from build123d import *

# Parameters (mm, degrees)
F0_W     = 10
F0_H     = 31
F0_R     = 1.8
F1_DEPTH = 4
F0_H_2   = 3
F2_DEPTH = 19
F3_R     = 1.8
F4_DEPTH = 25
F5_R     = 2


with BuildPart() as f1:
    # F0 (on Front) → F1 (new body)
    with BuildSketch(Plane.XZ):
        with Locations((0.497756, 2.022149)):
            Rectangle(F0_W, F0_H)
        with Locations((0.497756, 13.522149)):
            Circle(F0_R, mode=Mode.SUBTRACT)
    extrude(amount=F1_DEPTH)

    # F0 (on Front) → F2 (join)
    with BuildSketch(Plane.XZ):
        with Locations((0.497756, -14.977851)):
            Rectangle(F0_W, F0_H_2)
    extrude(amount=F2_DEPTH)

    # F3 (on face) → F4 (cut)
    with BuildSketch(Plane.XY.offset(-13.477851)):
        with Locations((0.497756, -14)):
            Circle(F3_R)
    extrude(amount=-F4_DEPTH, mode=Mode.SUBTRACT)

    # F5
    f5_edges = [f1.edges().sort_by_distance(p)[0] for p in [
        (-4.502244, -2, 17.522149),
        (5.497756, -2, 17.522149),
        (5.497756, -19, -14.977851),
        (-4.502244, -19, -14.977851),
    ]]
    fillet(f5_edges, radius=F5_R)


solid = f1.part
Work out the finished part from the listing and answer in its coordinate system (mm). A direction names the side the tool comes from. Give positions to 0.01 mm unless a question says otherwise; leave off trailing zeros. Loops run counter-clockwise (first coordinate to the right, second up) from the corner with the lowest first, then second, coordinate; pieces in that order, holes last. Notation, with made-up numbers: M 52.5,48.25 L 80.5,48.25 A21 ccw 80.5,73.25 Z; hole C 54.25,76 d6. An arc over 180 degrees is marked long. Use CSV: the item, a comma, the result in double quotes.
1) Find section A-A on y = -14. Write down the section's boundary in (x, z), plus the area to 3 significant figures.
Answer:
outline,"M -4.5,-16.48 L -1.3,-16.48 L -1.3,-13.48 L -4.5,-13.48 Z; M 2.3,-16.48 L 5.5,-16.48 L 5.5,-13.48 L 2.3,-13.48 Z"
area,"19.2 mm^2"
2) Find section B-B on z = 12.5. Write down the section's boundary in (x, y).
Answer:
outline,"M -4.5,-4 L -0.98,-4 L -0.98,0 L -4.5,0 Z; M 1.98,-4 L 5.5,-4 L 5.5,0 L 1.98,0 Z"
3) Given P1, Ø5, axis at x = 2.5, y = -12, coming from the +Z side; P2, Ø2, axis at x = 0.5, y = -14, coming from the +Z side, each flat-ended and moving along its own axis, determine where each tip first touches the part or whether it passes through.
Answer:
P1,"z = -13.48"
P2,"through"
4) Which of the six approach directions +Z, -Z, +X, -X, +Y, -Y give full straight-line access (tool end or side, diameter ignored) to faces 4 (the flat face through (0, -4, 2)), 5 (the flat face through (0, 0, 1))?
Answer:
face 4,"+Z, +X, -X, -Y"
face 5,"+Z, -Z, +X, -X, +Y"
5) Determine the mould class of faces 1 (the cylindrical face through (0.263, -1.972, 15.307)), 2 (the flat face through (5.498, -3, -4)), 3 (the cylindrical face through (-3.93, -18.4, -14.96)) for opening direction X: released by +X, released by -X, zero draft, split by the parting line, or undercut.
Answer:
face 1,"undercut"
face 2,"released by +X"
face 3,"released by -X"
6) Consider L1, parallel to Z at x = -2.25, y = -9; L2, parallel to Y at x = -2.75, z = -8; L3, parallel to X at y = -3.5, z = 12.5. Determine where each line is inside the solid, lowest interval first.
Answer:
L1,"-16.48 to -13.48"
L2,"-4 to 0"
L3,"-4.5 to -0.98, 1.98 to 5.5"
7) Find section D-D on y = -2.5. Write down the section's boundary in (x, z), plus the area to 3 significant figures.
Answer:
outline,"M -4.5,-16.48 L 5.5,-16.48 L 5.5,15.52 A2 ccw 3.5,17.52 L -2.5,17.52 A2 ccw -4.5,15.52 Z; hole C 0.5,13.52 d3.6"
area,"328 mm^2"
8) Find section C-C on x = 1.5. Write down the section's boundary in (y, z), plus the area to 3 significant figures.
Answer:
outline,"M -19,-16.48 L -15.5,-16.48 L -15.5,-13.48 L -19,-13.48 Z; M -12.5,-16.48 L 0,-16.48 L 0,12.03 L -4,12.03 L -4,-13.48 L -12.5,-13.48 Z; M -4,15.02 L 0,15.02 L 0,17.52 L -4,17.52 Z"
area,"160 mm^2"
